from build123d import *

# Parameters (mm, degrees)
F0_R     = 10
F1_DEPTH = 30
F2_R     = 5
F3_DEPTH = 10


with BuildPart() as f1:
    # F0 (on Top) → F1 (new body)
    with BuildSketch(Plane.XY):
        Polygon((15, 30), (-15, 30), (-15, -30), (0, -30), (15, -30), align=None)
        Circle(F0_R, mode=Mode.SUBTRACT)
        Polygon((0, -30), (-15, -30), (-5, -45), (0, -45), align=None)
        Polygon((5, -45), (15, -30), (0, -30), (0, -45), align=None)
        Circle(F0_R)
    extrude(amount=F1_DEPTH)

    # F2
    f2_edges = [f1.edges().sort_by_distance(p)[0] for p in [
        (15, 0, 0),
        (-15, 0, 0),
        (-15, 0, 30),
        (15, 0, 30),
        (-10, -37.5, 30),
        (10, -37.5, 30),
        (-5, -45, 15),
        (5, -45, 15),
        (0, -45, 0),
        (0, -45, 30),
        (10, -37.5, 0),
        (-10, -37.5, 0),
    ]]
    fillet(f2_edges, radius=F2_R)

    # F0 (on Top) → F3 (cut)
    with BuildSketch(Plane.XY):
        Circle(F0_R)
    extrude(amount=F3_DEPTH, mode=Mode.SUBTRACT)


solid = f1.part
Could you check a few things on this model? Use its own coordinates, in mm. Give positions to 0.01 mm unless a question says otherwise; leave off trailing zeros. Order: outer loops, then holes, each group sorted by start corner. A loop starts at its lowest first (then second) coordinate and runs counter-clockwise, first axis right, second up. Notation, with made-up numbers: (45, 24) -> (49, 24) arc R32 ccw to (49, 58) -> close; hole circle Ø10 at (27, 64.25). An arc over 180 degrees is marked (long way). Return JSON: item names as keys, results as strings.
1. Imagine slicing it at D-D on z = 12.5. List the corners of the cut face in (x, y) for me.
Answer list:
{"outline": "(-15, -30) -> (-6.48, -42.77) arc R5 ccw to (-2.32, -45) -> (2.32, -45) arc R5 ccw to (6.48, -42.77) -> (15, -30) -> (15, 30) -> (-15, 30) -> close"}
2. Imagine slicing it at B-B on x = 0. List the corners of the cut face in (y, z) for me.
Answer list:
{"outline": "(-45, 5) arc R5 ccw to (-40, 0) -> (-10, 0) -> (-10, 10) -> (10, 10) -> (10, 0) -> (30, 0) -> (30, 30) -> (-40, 30) arc R5 ccw to (-45, 25) -> close"}
3. Imagine slicing it at A-A on z = 8. List the corners of the cut face in (x, y) for me.
Answer list:
{"outline": "(-15, -30) -> (-6.48, -42.77) arc R5 ccw to (-2.32, -45) -> (2.32, -45) arc R5 ccw to (6.48, -42.77) -> (15, -30) -> (15, 30) -> (-15, 30) -> close; hole circle Ø20 at (0, 0)"}
4. Imagine slicing it at C-C on y = 24.5. List the corners of the cut face in (x, z) for me.
Answer list:
{"outline": "(-15, 5) arc R5 ccw to (-10, 0) -> (10, 0) arc R5 ccw to (15, 5) -> (15, 25) arc R5 ccw to (10, 30) -> (-10, 30) arc R5 ccw to (-15, 25) -> close"}
5. Thinking about a two-plate mould opening in X: for faces 1 (the cylindrical face through (14, 0, 2)), 2 (the cylindrical face through (-9.496, -35.685, 1.504)), 3 (the flat face through (0, 30, 15)), 4 (the cylindrical face through (-2.17, -9.76, 4.93)), which applies, pulls with the +X half, pulls with the -X half, needs draft (parallel to the pull), parting line crosses it, or undercut?
Answer list:
{"face 1": "pulls with the +X half", "face 2": "pulls with the -X half", "face 3": "needs draft", "face 4": "undercut"}
6. I need wall thicknesses on line 1 (Y direction, x = 0, z = 7.75); line 2 (X direction, y = 0, z = 6); line 3 (Z direction, x = 9.5, y = -3). Which ranges of each line are inside material? Lowest first, please. Write a range as from..to.
Answer list:
{"line 1": "y = -45..-10, 10..30", "line 2": "x = -15..-10, 10..15", "line 3": "z = 10..30"}
7. For pin 1 Ø2 at (x, y) = (7, -35.5) entering from +Z, with a flat end and sliding along its axis, tell me the tip position at first contact or that it passes through.
Answer list:
{"pin 1": "stops at z = 29.98"}
